Can you work these out from the model? Positions are in its coordinate system, mm. A direction names the side the tool comes from. Coordinates: 2 decimals unless noted, no trailing zeros. Order: outer loops, then holes, each group sorted by start corner. A loop starts at its lowest first (then second) coordinate and runs counter-clockwise, first axis right, second up. Notation, with made-up numbers: (-11.5, 10) -> (10.5, 10) arc R20 ccw to (10.5, 25) -> close; hole circle Ø8 at (3, 85.25). An arc over 180 degrees is marked (long way). Answer in a Markdown table with one row per item.
Autodesk Inventor part; units mm, degrees
ref_plane "Work Plane1" through (-31.7062, 85.6066, -5) normal (0, 0, 1) x (1, 0, 0)
ref_plane "YZ Plane" through (0, 0, 0) normal (1, 0, 0) x (0, 1, 0)
ref_plane "XZ Plane" through (0, 0, 0) normal (0, 1, 0) x (-1, 0, 0)
sketch "Sketch1" plane through (0, 0, 0) normal (0, 0, 1) x (1, 0, 0)
  line L0 (-201.7062, 85.6066) -> (-31.7062, 85.6066)
  line L1 (-31.7062, 85.6066) -> (-31.7062, 33.6066)
  line L2 (-31.7062, 33.6066) -> (-201.7062, 33.6066)
  line L3 (-201.7062, 33.6066) -> (-201.7062, 85.6066)
  line L4 (-36.7062, 80.6066) -> (-196.7062, 80.6066)
  line L5 (-196.7062, 38.6066) -> (-36.7062, 38.6066)
  line L6 (-196.7062, 59.6066) -> (-36.7062, 59.6066)
  line L7 (-36.7062, 65.0934) -> (-196.7062, 65.0934)
  line L8 (-36.7062, 38.6066) -> (-36.7062, 59.6066)
  line L9 (-36.7062, 65.0934) -> (-36.7062, 80.6066)
  line L10 (-196.7062, 80.6066) -> (-196.7062, 65.0934)
  line L11 (-196.7062, 59.6066) -> (-196.7062, 38.6066)
  line L12 (-196.7062, 80.6066) -> (-201.7062, 80.6066)
  line L13 (-36.7062, 80.6066) -> (-31.7062, 80.6066)
  line L14 (-36.7062, 80.6066) -> (-36.7062, 85.6066)
  line L15 (-36.7062, 38.6066) -> (-36.7062, 33.6066)
  line L16 (-36.7062, 38.6066) -> (-31.7062, 38.6066)
  line L17 (-196.7062, 38.6066) -> (-201.7062, 38.6066)
  line L18 (-196.7062, 38.6066) -> (-196.7062, 33.6066)
  line L19 (-196.7062, 80.6066) -> (-196.7062, 85.6066)
  circle A0 centre (-199.2062, 83.1066) radius 2.5
  circle A1 centre (-199.2062, 36.1066) radius 2.5
  circle A2 centre (-34.2062, 36.1066) radius 2.5
  circle A3 centre (-34.2062, 72.6066) radius 2.5
  point P0 (0, 0)
extrude "Extrusion1" add sketch "Sketch1" against normal blind 5 contours L19 A0 L0 | L0 L14 L4 L19 | L0 L1 L13 L14 | A0 L3 L0 | A0 | L19 L12 A0 | L13 L1 A3 L9 | A0 L12 L3 | L10 L7 L9 A3 L1 L16 L8 L6 L11 L17 L3 L12 | A3 | L17 A1 L3 | L1 A2 L16 | A1 L2 L3 | A1 | L17 L18 A1 | A2 | L1 L2 A2 | A2 L15 L16 | A1 L18 L2 | L5 L15 L2 L18 | L2 L15 A2
ref_plane "Work Plane1" through (-31.7062, 85.6066, -5) normal (0, 0, 1) x (1, 0, 0)
sketch "Sketch2" plane through (0, 0, -5) normal (0, 0, -1) x (-1, 0, 0)
  line L0 (36.7062, 65.0934) -> (196.7062, 65.0934)
  line L1 (196.7062, 65.0934) -> (196.7062, 59.6066)
  line L2 (196.7062, 59.6066) -> (36.7062, 59.6066)
  line L3 (36.7062, 59.6066) -> (36.7062, 65.0934)
  point P0 (0, 0)
extrude "Extrusion2" cut sketch "Sketch2" against normal blind 1
hole "Hole1" at (-199.2062, 83.1066, 0) direction (0, 0, -1) diameter 3 depth 5 tip angle 118
hole "Hole2" at (-199.2062, 36.1066, 0) direction (0, 0, -1) diameter 3 depth 5 tip angle 118
hole "Hole4" at (-34.2062, 36.1066, 0) direction (0, 0, -1) diameter 3 depth 5 tip angle 118
hole "Hole5" at (-34.2062, 72.6066, 0) direction (0, 0, -1) diameter 3 depth 5 tip angle 118
thread "Thread1"
thread "Thread2"
thread "Thread3"
thread "Thread4"
properties part number "lateral suport"
(1) Suppose I cut it at D-D (y = 62.5). Please give me the cut outline in (x, z).
Response values:
| item | result |
|---|---|
| outline | (-201.71, -5) -> (-196.71, -5) -> (-196.71, -4) -> (-36.71, -4) -> (-36.71, -5) -> (-31.71, -5) -> (-31.71, 0) -> (-201.71, 0) -> close |
(2) Suppose I cut it at A-A (y = 50). Please give me the cut outline in (x, z), and give its area (3 significant figures).
Response values:
| item | result |
|---|---|
| outline | (-201.71, -5) -> (-196.71, -5) -> (-196.71, 0) -> (-201.71, 0) -> close; (-36.71, -5) -> (-31.71, -5) -> (-31.71, 0) -> (-36.71, 0) -> close |
| area | 50.0 mm2 |
(3) On a 3-axis mill with a long thin cutter (end or side, diameter ignored), from which of +Z, -Z, +X, -X, +Y, -Y can I reach the whole of each face in a straight line? I mean faces 4 (the flat face through (-118, 85.607, -2)), 5 (the flat face through (-118, 59.607, -2)), 6 (the flat face through (-116, 62, -4)). Say none if no direction works.
Response values:
| item | result |
|---|---|
| face 4 | +Z, -Z, +X, -X, +Y |
| face 5 | +Z, -Z |
| face 6 | -Z |
(4) I need wall thicknesses on line 1 (Y direction, x = -103.5, z = -2.75); line 2 (X direction, y = 36, z = -3.7); line 3 (Y direction, x = -61, z = -4.75). Which ranges of each line are inside material? Lowest first, please. Write a range as [from, to].
Response values:
| item | result |
|---|---|
| line 1 | [33.61, 38.61], [59.61, 65.09], [80.61, 85.61] |
| line 2 | [-201.71, -200.7], [-197.71, -35.7], [-32.71, -31.71] |
| line 3 | [33.61, 38.61], [80.61, 85.61] |
(5) Suppose I cut it at C-C (z = -3.15). Please give me the cut outline in (x, y).
Response values:
| item | result |
|---|---|
| outline | (-201.71, 33.61) -> (-31.71, 33.61) -> (-31.71, 85.61) -> (-201.71, 85.61) -> close; hole circle Ø3 at (-199.21, 36.11); hole circle Ø3 at (-199.21, 83.11); hole (-196.71, 38.61) -> (-36.71, 38.61) -> (-36.71, 59.61) -> (-196.71, 59.61) -> close; hole (-196.71, 65.09) -> (-36.71, 65.09) -> (-36.71, 80.61) -> (-196.71, 80.61) -> close; hole circle Ø3 at (-34.21, 36.11); hole circle Ø3 at (-34.21, 72.61) |
(6) Will this pin go through, and if not, where does the flat tip stop? pin 1 Ø6 at (x, y) = (-135.5, 61.5) entering from -Z.
Response values:
| item | result |
|---|---|
| pin 1 | z = -4 |
(7) We'd pull the mould along X, two halves only. Please class faces 1 (the flat face through (-111, 60, 0)), 2 (the cylindrical face through (-200.693, 83.302, -2.535)), 3 (the flat face through (-201.706, 59, -2)): +X half, -X half, draft (parallel to the pull), parting line (faces both ways), or undercut.
Response values:
| item | result |
|---|---|
| face 1 | draft |
| face 2 | undercut |
| face 3 | -X half |
(8) Suppose I cut it at B-B (x = -181). Please give me the cut outline in (y, z).
Response values:
| item | result |
|---|---|
| outline | (33.61, -5) -> (38.61, -5) -> (38.61, 0) -> (33.61, 0) -> close; (59.61, -4) -> (65.09, -4) -> (65.09, 0) -> (59.61, 0) -> close; (80.61, -5) -> (85.61, -5) -> (85.61, 0) -> (80.61, 0) -> close |
